from build123d import *

# Parameters (mm, degrees)
F0_W      = 50.8
F0_H      = 50.8
F1_DEPTH  = 76.2
F2_DEPTH  = 25.4
F3_R      = 12.7
F4_DEPTH  = 25.4
F5_DEPTH  = 25.4
F6_W      = 25.4
F6_H      = 25.4
F7_DEPTH  = 25.4
F8_DEPTH  = 25.4
F9_DEPTH  = 25.4
F10_R     = 12.7
F11_DEPTH = 25.4


with BuildPart() as f1:
    # F0 (on Front) → F1 (new body)
    with BuildSketch(Plane.XZ):
        with Locations((-25.4, 25.4)):
            Rectangle(F0_W, F0_H)
    extrude(amount=F1_DEPTH)

    # F2 (cut): a face of the model
    f2_faces = [f1.faces().sort_by_distance(p)[0] for p in [
        (-25.4, -76.2, 25.4),
    ]]
    extrude(f2_faces, amount=-F2_DEPTH, mode=Mode.SUBTRACT)

    # F3 (on face) → F4 (cut)
    with BuildSketch(Plane.XY.offset(50.8)):
        with Locations((-25.7175005972, -26.3298209757)):
            Circle(F3_R)
    extrude(amount=-F4_DEPTH, mode=Mode.SUBTRACT)

    # F5 (add): a face of the model
    f5_faces = [f1.faces().sort_by_distance(p)[0] for p in [
        (-25.4, -50.8, 25.4),
    ]]
    extrude(f5_faces, amount=F5_DEPTH)

    # F6 (on face) → F7 (join)
    with BuildSketch(Plane.XZ.offset(76.2)):
        with Locations((-25.6721441031, 25.1505357817)):
            Rectangle(F6_W, F6_H)
    extrude(amount=F7_DEPTH)

    # F8 (cut): a face of the model
    f8_faces = [f1.faces().sort_by_distance(p)[0] for p in [
        (-25.4, -76.2, 0.7184204897),
    ]]
    extrude(f8_faces, amount=-F8_DEPTH, mode=Mode.SUBTRACT)

    # F9 (cut): a face of the model
    f9_faces = [f1.faces().sort_by_distance(p)[0] for p in [
        (-25.6721441031, -101.6, 25.1505357817),
    ]]
    extrude(f9_faces, amount=-F9_DEPTH, mode=Mode.SUBTRACT)

    # F10 (on face) → F11 (join)
    with BuildSketch(Plane.YZ):
        with Locations((-25.7175005972, 24.9010715634)):
            Circle(F10_R)
    extrude(amount=F11_DEPTH)


solid = f1.part
Here's how the part is built. I have some questions about the finished solid (model axes, mm). A direction names the side the tool comes from. Round coordinates to 2 decimals unless told otherwise and drop trailing zeros. Order: outer loops, then holes, each group sorted by start corner. A loop starts at its lowest first (then second) coordinate and runs counter-clockwise, first axis right, second up. Notation, with made-up numbers: (48, 52) -> (54, 52) arc R16 ccw to (54, 58) -> close; hole circle Ø2 at (-39.75, -38). An arc over 180 degrees is marked (long way). Return JSON: item names as keys, results as strings.
Q1. If we section it at B-B on x = -31: List the corners of the cut face in (y, z) for me.
Filled sheet:
{"outline": "(-76.2, 12.45) -> (-50.8, 12.45) -> (-50.8, 0) -> (0, 0) -> (0, 50.8) -> (-14.78, 50.8) -> (-14.78, 25.4) -> (-37.88, 25.4) -> (-37.88, 50.8) -> (-50.8, 50.8) -> (-50.8, 37.85) -> (-76.2, 37.85) -> close"}
Q2. If we mould it in two halves opening along Y, with no side actions, what happens to faces 1 (the flat face through (-26, 0, 26)), 2 (the cylindrical face through (12.522, -28.471, 12.503)), 3 (the flat face through (-26, -26, 25.4))? For each: released by +Y, released by -Y, zero draft, split by the parting line, or undercut.
Filled sheet:
{"face 1": "released by +Y", "face 2": "split by the parting line", "face 3": "undercut"}
Q3. If we section it at D-D on x = -3: List the corners of the cut face in (y, z) for me.
Filled sheet:
{"outline": "(-50.8, 0) -> (0, 0) -> (0, 50.8) -> (-50.8, 50.8) -> close"}
Q4. For pin 1 Ø3 at (x, y) = (-37, -48) entering from -Z; pin 2 Ø7.5 at (y, z) = (-64, 19.5) entering from -X; pin 3 Ø7.5 at (y, z) = (-62.5, 29) entering from +X; pin 4 Ø6 at (y, z) = (-35.5, 5) entering from +X, each with a flat end and sliding along its axis, tell me the tip position at first contact or that it passes through.
Filled sheet:
{"pin 1": "stops at z = 0", "pin 2": "stops at x = -38.37", "pin 3": "stops at x = -12.97", "pin 4": "stops at x = 0"}
Q5. If we section it at C-C on y = -35: List the corners of the cut face in (x, z) for me.
Filled sheet:
{"outline": "(-50.8, 0) -> (0, 0) -> (0, 16.23) -> (25.4, 16.23) -> (25.4, 33.57) -> (0, 33.57) -> (0, 50.8) -> (-16.44, 50.8) -> (-16.44, 25.4) -> (-35, 25.4) -> (-35, 50.8) -> (-50.8, 50.8) -> close"}
Q6. I need wall thicknesses on line 1 along X through (y, z) = (-40.5, 8.5); line 2 along X through (y, z) = (-18, 27). Which ranges of each line are inside material? Lowest first, please. Write a range as from..to.
Filled sheet:
{"line 1": "x = -50.8..0", "line 2": "x = -50.8..-35.3, -16.13..25.4"}
Q7. If we section it at A-A on z = 32.5: List the corners of the cut face in (x, y) for me, plus the area to 3 significant figures.
Filled sheet:
{"outline": "(-50.8, -50.8) -> (-38.37, -50.8) -> (-38.37, -76.2) -> (-12.97, -76.2) -> (-12.97, -50.8) -> (0, -50.8) -> (0, -35.89) -> (25.4, -35.89) -> (25.4, -15.54) -> (0, -15.54) -> (0, 0) -> (-50.8, 0) -> close; hole circle Ø25.4 at (-25.72, -26.33)", "area": "3,240 mm^2"}
Q8. Which directions (+Z, -Z, +X, -X, +Y, -Y) give clear straight access to the entire face, cutting with the end or side of a thin tool? Please do faces 4 (the cylindrical face through (-27.371, -13.738, 38.278)), 5 (the flat face through (-26, -64, 37.851)), 6 (the flat face through (-26, -64, 12.451)), 7 (the flat face through (-12.972, -64, 25)).
Filled sheet:
{"face 4": "+Z", "face 5": "+Z, +X, -X, -Y", "face 6": "-Z, +X, -X, -Y", "face 7": "+Z, -Z, +X, -Y"}
